Build history of the part. All positions in model axes, mm. Face numbers are marked on the shaded views. Give positions to 0.01 mm unless a question says otherwise; leave off trailing zeros. Loops run counter-clockwise (first coordinate to the right, second up) from the corner with the lowest first, then second, coordinate; pieces in that order, holes last. Notation, with made-up numbers: M -28,75 L -24,75 A22 cw -24,91 Z; hole C 33.25,25.25 d3. An arc over 180 degrees is marked long. Answer as a JSON object with one key per item and string values. Group by question number.
1. Slice it at D-D (z = -89). List the corners of the cut face in (x, y), then the cut area to 3 significant figures.
2. Slice it at C-C (y = 5.25). List the corners of the cut face in (x, z), then the cut area to 3 significant figures.
3. Slice it at B-B (x = 50). List the corners of the cut face in (y, z).
4. Slice it at A-A (z = 0). List the corners of the cut face in (x, y).
5. Drill centre lines: line 1 along X through (y, z) = (7.5, 0); line 2 along Z through (x, y) = (-64, 8); line 3 along Z through (x, y) = (54.5, 2.75). Where is each one in solid material? Low to high. Write a range as [from, to].
6. Mould opens along Y. For the marked faces 1 and 2 say: released by +Y, released by -Y, zero draft, split by the parting line, or undercut.
7. Drop flat-ended pins along their axis: pin 1 Ø2 at (y, z) = (9.5, -74) entering from -X; pin 2 Ø6 at (x, y) = (15.5, 5.5) entering from -Z; pin 3 Ø6 at (y, z) = (7.5, 99.5) entering from -X. Give the stop position or say it passes through.
from build123d import *

# Parameters (mm, degrees)
SKETCH1_R                = 105
SKETCH1_R_2              = 80
BOSS_EXTRUDE1_DEPTH      = 12.7
CUT_EXTRUDE1_DEPTH       = 150.034526201
FILLET1_R                = 1
CIRPATTERN1_COUNT        = 3
FILLET1_OF_CIRPATTERN1_R = 1


with BuildPart() as part:
    # Sketch1 → Boss-Extrude1 (new body)
    with BuildSketch(Plane(origin=(0, 0, 0), x_dir=(1, 0, 0), z_dir=(0, 1, 0))):
        with Locations(Location((0, 0, 0), (0, 0, 270))):
            Circle(SKETCH1_R)
        with Locations(Location((0, 0, 0), (0, 0, 270))):
            Circle(SKETCH1_R_2, mode=Mode.SUBTRACT)
    extrude(amount=BOSS_EXTRUDE1_DEPTH)

    # Sketch2 → Cut-Extrude1 (cut, through all)
    with BuildSketch(Plane(origin=(0, 12.7, 0), x_dir=(1, 0, 0), z_dir=(0, 1, 0))):
        with BuildLine():
            Line((6.35, -105), (-6.35, -105))
            Line((-6.35, -105), (-6.35, -96.4))
            ThreePointArc((-6.35, -96.4), (-9.55, -93.2), (-6.35, -90))
            Line((-6.35, -90), (6.35, -90))
            ThreePointArc((6.35, -90), (9.55, -93.2), (6.35, -96.4))
            Line((6.35, -96.4), (6.35, -105))
        make_face()
    cut_extrude1 = extrude(amount=-CUT_EXTRUDE1_DEPTH, mode=Mode.SUBTRACT)

    # Fillet1
    fillet1_edges = [part.edges().sort_by_distance(p)[0] for p in [
        (6.35, 6.35, 96.4),
        (-6.35, 6.35, 96.4),
    ]]
    fillet(fillet1_edges, radius=FILLET1_R)

    # CirPattern1: Cut-Extrude1 ×3 about axis
    cirpattern1_axis = Axis((0, 0, 0), (0, 1, 0))
    for i in range(1, CIRPATTERN1_COUNT):
        add(cut_extrude1.rotate(cirpattern1_axis, i * 360 / CIRPATTERN1_COUNT), mode=Mode.SUBTRACT)

    # Fillet1 of CirPattern1
    fillet1_of_cirpattern1_edges = [part.edges().sort_by_distance(p)[0] for p in [
        (80.309848925, 6.35, -53.699261314),
        (86.659848925, 6.35, -42.700738686),
        (-86.659848925, 6.35, -42.700738686),
        (-80.309848925, 6.35, -53.699261314),
    ]]
    fillet(fillet1_of_cirpattern1_edges, radius=FILLET1_OF_CIRPATTERN1_R)


solid = part.part
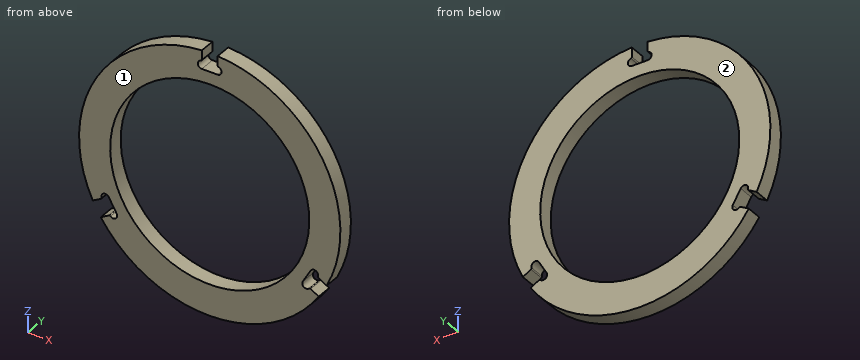
Established:
{
 "1": {"outline": "M -55.71,0 L 55.71,0 L 55.71,12.7 L -55.71,12.7 Z", "area": "1,420 mm^2"},
 "2": {"outline": "M -93.94,-46.9 L -87.42,-43.14 A1 ccw -86.96,-41.99 A3.2 cw -81.12,-39.5 L -74.77,-50.5 A3.2 cw -79.85,-54.31 A1 ccw -81.07,-54.14 L -87.59,-57.9 A105 ccw 87.59,-57.9 L 81.07,-54.14 A1 ccw 79.85,-54.31 A3.2 cw 74.77,-50.5 L 81.12,-39.5 A3.2 cw 86.96,-41.99 A1 ccw 87.42,-43.14 L 93.94,-46.9 A105 ccw 6.35,104.81 L 6.35,97.28 A1 ccw 7.11,96.31 A3.2 cw 6.35,90 L -6.35,90 A3.2 cw -7.11,96.31 A1 ccw -6.35,97.28 L -6.35,104.81 A105 ccw Z; hole C 0,0 d160", "area": "13,900 mm^2"},
 "3": {"outline": "M 0,-92.33 L 12.7,-92.33 L 12.7,-62.45 L 0,-62.45 Z; M 0,62.45 L 12.7,62.45 L 12.7,92.33 L 0,92.33 Z"},
 "4": {"outline": "M -105,0 L -80,0 L -80,12.7 L -105,12.7 Z; M 80,0 L 105,0 L 105,12.7 L 80,12.7 Z"},
 "5": {"line 1": "x = [-105, -80], [80, 105]", "line 2": "z = [-83.24, -48], [48, 83.24]", "line 3": "z = [-89.75, -58.56], [58.56, 89.75]"},
 "6": {"face 1": "released by -Y", "face 2": "released by +Y"},
 "7": {"pin 1": "stops at x = -75.47", "pin 2": "stops at z = -104.25", "pin 3": "stops at x = -41.39"}
}
